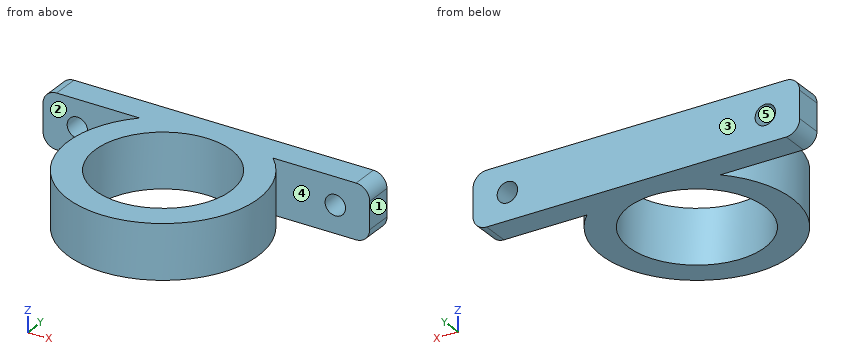
from build123d import *

# Parameters (mm, degrees)
CROQUIS1_R              = 10
SALIENTE_EXTRUIR1_DEPTH = 8
REDONDEO1_R             = 2
CROQUIS2_R              = 1.5
CORTAR_EXTRUIR1_DEPTH   = 35.871191548


with BuildPart() as part:
    # Croquis1 → Saliente-Extruir1 (new body)
    with BuildSketch(Plane.XY):
        with BuildLine():
            Line((0, 14), (24, 14))
            Line((24, 14), (24, 10))
            Line((24, 10), (9.797958971, 10))
            ThreePointArc((9.797958971, 10), (0, -14), (-9.797958971, 10))
            Line((-9.797958971, 10), (-24, 10))
            Line((-24, 10), (-24, 14))
            Line((-24, 14), (0, 14))
        make_face()
        Circle(CROQUIS1_R, mode=Mode.SUBTRACT)
    extrude(amount=SALIENTE_EXTRUIR1_DEPTH)

    # Redondeo1
    redondeo1_edges = [part.edges().sort_by_distance(p)[0] for p in [
        (24, 12, 8),
        (-24, 12, 8),
        (-24, 12, 0),
        (24, 12, 0),
    ]]
    fillet(redondeo1_edges, radius=REDONDEO1_R)

    # Croquis2 → Cortar-Extruir1 (cut, through all)
    with BuildSketch(Plane.XZ.offset(-10)):
        with Locations(Location((-18.949489743, 4, 0), (0, 0, 270))):
            Circle(CROQUIS2_R)
        with Locations(Location((18.949489743, 4, 0), (0, 0, 270))):
            Circle(CROQUIS2_R)
    extrude(amount=-CORTAR_EXTRUIR1_DEPTH, mode=Mode.SUBTRACT)


solid = part.part
The model under review builds one solid part; all positions refer to its coordinate system, in mm. Face numbers are marked on the shaded views. A direction names the side the tool comes from. Give positions to 0.01 mm unless a question says otherwise; leave off trailing zeros. Order: outer loops, then holes, each group sorted by start corner. A loop starts at its lowest first (then second) coordinate and runs counter-clockwise, first axis right, second up. Notation, with made-up numbers: M 27,20.25 L 56,20.25 A12 cw 56,43.25 Z; hole C 51,-1.5 d7. An arc over 180 degrees is marked long. Answer in a Markdown table with one row per item. Add a question column.
1. Add section B-B on z = 4. State the section outline as (x, y) points.
2. For pin 1 Ø1.5 at (y, z) = (-6.5, 3) entering from -X; pin 2 Ø4 at (x, z) = (-18.95, 4) entering from -Y, all flat-tipped, find the tip position at first contact; note any pin that passes through.
3. Machinability: for the marked faces 4 and 5, which of the approach directions +Z, -Z, +X, -X, +Y, -Y give a long, thin tool a straight path to every point of the face, cutting with its end or side? Answer none if there is none.
4. Add section A-A on x = 0. State the section outline as (y, z) points, plus the area to 3 significant figures.
5. Add section D-D on z = 0.5. State the section outline as (x, y) points, plus the area to 3 significant figures.
6. Mouldability with a two-part tool opening along Y and no side actions: class the marked faces 1, 2 and 3 as released by +Y, released by -Y, zero draft, split by the parting line, or undercut.
7. To check wall thickness, follow line 1 along X through (y, z) = (12.45, 4); line 2 along Y through (x, z) = (-1.5, 6.5); line 3 along Z through (x, y) = (18, 12.75). State the ranges of each line that lie inside material, in increasing order.
The answers:
| question | item | result |
|---|---|---|
| 1 | outline | M -24,10 L -20.45,10 L -20.45,14 L -24,14 Z; M -17.45,10 L -9.8,10 A14 ccw long 9.8,10 L 17.45,10 L 17.45,14 L -17.45,14 Z; M 20.45,10 L 24,10 L 24,14 L 20.45,14 Z; hole C 0,0 d20 |
| 2 | pin 1 | x = -12.76 |
| 2 | pin 2 | y = 10 |
| 3 | face 4 | +Z, -Z, +X |
| 3 | face 5 | +Y, -Y |
| 4 | outline | M -14,0 L -10,0 L -10,8 L -14,8 Z; M 10,0 L 14,0 L 14,8 L 10,8 Z |
| 4 | area | 64.0 mm2 |
| 5 | outline | M -23.32,10 L -9.8,10 A14 ccw long 9.8,10 L 23.32,10 L 23.32,14 L -23.32,14 Z; hole C 0,0 d20 |
| 5 | area | 434 mm2 |
| 6 | face 1 | zero draft |
| 6 | face 2 | undercut |
| 6 | face 3 | released by +Y |
| 7 | line 1 | -24 to -20.45, -17.45 to 17.45, 20.45 to 24 |
| 7 | line 2 | -13.92 to -9.89, 9.89 to 14 |
| 7 | line 3 | 0 to 2.84, 5.16 to 8 |
